Check sheet for the modelled part. Datum: model origin and axes. Units: mm. A direction names the side the tool comes from. Coordinates: 2 decimals unless noted, no trailing zeros. Write each loop counter-clockwise with the first axis right and the second up, starting at its lowest first coordinate (ties: lowest second). Pieces come first, ordered by that corner, then holes. Notation, with made-up numbers: M 46.25,-0.5 L 77.25,-0.5 A16 ccw 77.25,15.5 Z; hole C 1.25,34.25 d5. An arc over 180 degrees is marked long. Answer as CSV lines item,"result". Start each with the question number.
Q1. Sectioned sample at A-A, the plane z = 0. Record the cut outline in (x, y), then the cut area to 3 significant figures.
Q2. Access from +Z, -Z, +X, -X, +Y, -Y to the whole of each face (thin tool, end or side, straight path). Record for faces 1 (the flat face through (1.8, 8, 0)), 2 (the flat face through (1, 10, -1)).
Q3. Sectioned sample at B-B, the plane x = 0. Record the cut outline in (y, z), then the cut area to 3 significant figures.
Q4. Sectioned sample at D-D, the plane y = 7.25. Record the cut outline in (x, z).
Q5. Depth check by flat-ended pin: pin 1 Ø1.5 at (y, z) = (5.5, -1) entering from +X; pin 2 Ø1 at (y, z) = (8, -1) entering from -X; pin 3 Ø2.5 at (x, z) = (0, 0) entering from -Y. Enter the tip coordinate at first touch or a pass-through.
Q6. Mould release check, pull along Z, two halves, no side actions. Record for faces 3 (the flat face through (-1.8, 8, 0)), 4 (the cylindrical face through (0.466, 3.944, -1.478)), 5 (the cylindrical face through (0, 9, 1)), 6 (the cylindrical face through (0.1, 3.8, -2.6)): pulls with the +Z half, pulls with the -Z half, needs draft (parallel to the pull), parting line crosses it, or undercut.
Q7. Thickness scan on line 1 along X through (y, z) = (4, 0); line 2 along Z through (x, y) = (0, 9.5); line 3 along Y through (x, z) = (-1.85, -1.1). Record the ranges inside material, lowest first. Write a range as from..to.
Q8. Sectioned sample at C-C, the plane y = 9. Record the cut outline in (x, z), then the cut area to 3 significant figures.
from build123d import *

# Parameters (mm, degrees)
SKETCH1_R                 = 2.6
BOSS_EXTRUDE1_DEPTH       = 10
CUT_EXTRUDE1_START        = -3.2
CUT_EXTRUDE1_DEPTH        = 3.2
F_1_0MM_DOWEL_HOLE1_D     = 2
F_1_0MM_DOWEL_HOLE1_DEPTH = 3.399139381
F_1_0MM_DOWEL_HOLE1_TIP   = 0.600860619
SKETCH5_R                 = 1.55
CUT_EXTRUDE2_DEPTH        = 8


with BuildPart() as part:
    # Sketch1 → Boss-Extrude1 (new body)
    with BuildSketch(Plane(origin=(0, 0, 0), x_dir=(1, 0, 0), z_dir=(0, 1, 0))):
        with Locations(Location((0, 0, 0), (0, 0, 270))):
            Circle(SKETCH1_R)
    extrude(amount=BOSS_EXTRUDE1_DEPTH)

    # Sketch2 → Cut-Extrude1 (cut)
    with BuildSketch(Plane(origin=(0, 10, 0), x_dir=(1, 0, 0), z_dir=(0, 1, 0)).offset(CUT_EXTRUDE1_START)):
        with BuildLine():
            Line((-1.8, 1.876166304), (-1.8, -1.876166304))
            ThreePointArc((-1.8, -1.876166304), (-2.6, 0), (-1.8, 1.876166304))
        make_face()
        with BuildLine():
            Line((1.8, 1.876166304), (1.8, -1.876166304))
            ThreePointArc((1.8, -1.876166304), (2.6, 0), (1.8, 1.876166304))
        make_face()
    extrude(amount=CUT_EXTRUDE1_DEPTH, mode=Mode.SUBTRACT)

    # 1.0mm Dowel Hole1
    with Locations(Plane(origin=(0, 10, 0), x_dir=(1, 0, 0), z_dir=(0, 1, 0))):
        with Locations((0, 0)):
            Hole(F_1_0MM_DOWEL_HOLE1_D / 2, depth=F_1_0MM_DOWEL_HOLE1_DEPTH)
            with Locations((0, 0, -(F_1_0MM_DOWEL_HOLE1_DEPTH + F_1_0MM_DOWEL_HOLE1_TIP / 2))):  # 118° drill point
                Cone(0, F_1_0MM_DOWEL_HOLE1_D / 2, F_1_0MM_DOWEL_HOLE1_TIP, mode=Mode.SUBTRACT)

    # Sketch5 → Cut-Extrude2 (cut)
    with BuildSketch(Plane.XZ):
        with Locations(Location((0, 0, 0), (0, 0, 270))):
            Circle(SKETCH5_R)
    extrude(amount=-CUT_EXTRUDE2_DEPTH, mode=Mode.SUBTRACT)


solid = part.part
Output:
1,outline,"M -2.6,0 L -1.55,0 L -1.55,8 L -1,8 L -1,10 L -1.8,10 L -1.8,6.8 L -2.6,6.8 Z; M 1,8 L 1.55,8 L 1.55,0 L 2.6,0 L 2.6,6.8 L 1.8,6.8 L 1.8,10 L 1,10 Z"
1,area,"18.1 mm^2"
2,face 1,"+Z, -Z, +X, +Y"
2,face 2,"+Z, -Z, +X, -X, +Y"
3,outline,"M 0,-2.6 L 10,-2.6 L 10,-1 L 8,-1 L 8,-1.55 L 0,-1.55 Z; M 0,1.55 L 8,1.55 L 8,1 L 10,1 L 10,2.6 L 0,2.6 Z"
3,area,"23.2 mm^2"
4,outline,"M -1.8,-1.88 A2.6 ccw 1.8,-1.88 L 1.8,1.88 A2.6 ccw -1.8,1.88 Z; hole C 0,0 d3.1"
5,pin 1,"stops at x = 2.59"
5,pin 2,"stops at x = -1.8"
5,pin 3,"stops at y = 8"
6,face 3,"needs draft"
6,face 4,"undercut"
6,face 5,"undercut"
6,face 6,"parting line crosses it"
7,line 1,"x = -2.6..-1.55, 1.55..2.6"
7,line 2,"z = -2.6..-1, 1..2.6"
7,line 3,"y = 0..6.8"
8,outline,"M -1.8,-1.88 A2.6 ccw 1.8,-1.88 L 1.8,1.88 A2.6 ccw -1.8,1.88 Z; hole C 0,0 d2"
8,area,"14.0 mm^2"
